Autodesk Inventor part; units mm, degrees
ref_plane "YZ Plane" through (0, 0, 0) normal (1, 0, 0) x (0, 1, 0)
ref_plane "XZ Plane" through (0, 0, 0) normal (0, 1, 0) x (-1, 0, 0)
ref_plane "Arbeitsebene1" through (0, 0, -17.5) normal (0, 0, 1) x (1, 0, 0)
sketch "Skizze1" plane through (0, 0, -17.5) normal (0, 0, 1) x (1, 0, 0)
  arc A0 (5.2, -17) -> (15.2, -17) centre (10.2, -17) ccw
  circle A1 centre (10.2, -17) radius 2.3
  circle A2 centre (10.2, 22) radius 2.3
  arc A3 (15.2, 22) -> (5.2, 22) centre (10.2, 22) ccw
  line L0 (15.2, 22) -> (15.2, -17)
  line L1 (5.2, -17) -> (5.2, 22)
  point P0 (0, 0)
  dimension "d17" = 39
  dimension "d19" = 5
  dimension "d20" = 5
  dimension "d21" = 4.6
  dimension "d22" = 4.6
  dimension "d23" = 5.2
  dimension "d24" = 15.2
  dimension "d25" = 17
extrude "Extrusion1" add sketch "Skizze1" against normal blind 20
sketch "Skizze2" plane through (15.2, -17, -17.5) normal (1, 0, 0) x (0, 0, -1)
  circle A0 centre (0.5, 19.5) radius 16
  circle A1 centre (0.5, 19.5) radius 19
  line L0 (0, 44) -> (20, 44)
  line L1 (7, 44) -> (7, 37.3536)
  line L2 (7, 44) -> (4.49, 46.4189)
  line L3 (4.49, 46.4189) -> (-2.5421, 44.7897)
  line L4 (-2.5421, 44.7897) -> (-3.0105, 35.1101)
  line L5 (-3.09, 3.908) -> (-10.3297, -18.857)
  line L6 (-10.3297, -18.857) -> (9.5227, -24.4173)
  line L7 (9.5227, -24.4173) -> (7, -5)
  line L8 (0, -5) -> (20, -5)
  line L9 (7, -5) -> (7, 1.6464)
  line L10 (0, 0) -> (0, -5)
  line L11 (36.0228, 70.8555) -> (-22.3921, 70.8555)
  line L12 (-22.3921, 70.8555) -> (-22.3921, -28.3632)
  line L13 (-22.3921, -28.3632) -> (36.0228, -28.3632)
  line L14 (36.0228, -28.3632) -> (36.0228, 70.8555)
  point P0 (-17.5, 17)
  point P1 (-4.0018, 1.041)
  point P2 (-2.861, 38.2004)
  dimension "d5" = 3
  dimension "d6" = 7
  dimension "d26" = 49
  dimension "d27" = 24.5
  dimension "d28" = 32
  dimension "d29" = 18
extrude "Extrusion2" cut sketch "Skizze2" against normal blind 10 contours A0 | L14 L13 L12 L11
sketch "Skizze3" plane through (15.2, -17, -24.5) normal (0, 0, -1) x (-1, 0, 0)
  circle A0 centre (5, 39) radius 2.3
  line L0 (2.8638, 35.3) -> (0.7276, 39)
  line L1 (0.7276, 39) -> (2.8638, 42.7)
  line L2 (2.8638, 42.7) -> (7.1362, 42.7)
  line L3 (7.1362, 42.7) -> (9.2724, 39)
  line L4 (9.2724, 39) -> (7.1362, 35.3)
  line L5 (7.1362, 35.3) -> (2.8638, 35.3)
  line L6 (0.7276, 0) -> (2.8638, 3.7)
  line L7 (2.8638, 3.7) -> (7.1362, 3.7)
  line L8 (7.1362, 3.7) -> (9.2724, 0)
  line L9 (9.2724, 0) -> (7.1362, -3.7)
  line L10 (7.1362, -3.7) -> (2.8638, -3.7)
  line L11 (2.8638, -3.7) -> (0.7276, 0)
  point P0 (15.2, 17)
  point P1 (5, 0)
  point P2 (5, 0)
  point P3 (5.6446, 34.7922)
  point P4 (4.3554, 34.7922)
  dimension "d9" = 7.4
  dimension "d10" = 7.4
extrude "Extrusion3" cut sketch "Skizze3" along normal blind 10 and the other way blind 3.5 contours A0 | L0 L1 L2 L3 L4 L5 | L6 L7 L8 L9 L10 L11
fillet "Rundung1" radius 1 2 edges at (15.2, 2.5, -37) (5.2, 2.5, -37)
equation "\"d20\" = d19"
equation "\"d27\" = 0.5 * d26"
equation "\"d10\" = d9"
properties part number "Schelle32"
Here's how the part is built. I have some questions about the finished solid (model axes, mm). A direction names the side the tool comes from. Give positions to 0.01 mm unless a question says otherwise; leave off trailing zeros. Loops run counter-clockwise (first coordinate to the right, second up) from the corner with the lowest first, then second, coordinate; pieces in that order, holes last. Notation, with made-up numbers: M -11,64 L 21,64 A29 cw 21,100 Z; hole C 79,-11.75 d7. An arc over 180 degrees is marked long. Use one line per item in the form item = value. Start each with the question number.
Q1. I need wall thicknesses on line 1 along Y through (x, z) = (10.2, -18.5); line 2 along Y through (x, z) = (10.2, -19.25); line 3 along Y through (x, z) = (10.5, -30.5). Which ranges of each line are inside material? Lowest first, please.
Q2. Which directions (+Z, -Z, +X, -X, +Y, -Y) give clear straight access to the entire face, cutting with the end or side of a thin tool? Please do faces 1 (the flat face through (8, 24, -21)), 2 (the flat face through (15.2, 2.6, -34.2)).
Q3. If we section it at C-C (y = 2.5): Write out the boundary of the cut face in (x, z), then the cut area to 3 significant figures.
Q4. If we section it at D-D (x = 13): Write out the boundary of the cut face in (y, z).
Q5. Will these pins go through, and if not, where does the flat tip stop? pin 1 Ø4 at (x, y) = (9, 24.5) entering from -Z; pin 2 Ø6 at (x, z) = (14, -24) entering from +Y; pin 3 Ø2 at (y, z) = (12, -29) entering from +X; pin 4 Ø3.5 at (x, y) = (8, 21) entering from -Z.
Q6. If we section it at B-B (z = -20.25): Write out the boundary of the cut face in (x, y), then the cut area to 3 significant figures.
Taken from the geometry:
q1.line_1 = -22 to -19.3, -14.7 to -13.49, 18.49 to 19.7, 24.3 to 27
q1.line_2 = -22 to -19.3, -14.7 to -13.45, 18.45 to 19.7, 24.3 to 27
q1.line_3 = -11.81 to -7.49, 12.49 to 16.81
q2.face_1 = -Z
q2.face_2 = +Z, -Z, +X, +Y, -Y
q3.outline = M 5.2,-36 A1 ccw 6.2,-37 L 14.2,-37 A1 ccw 15.2,-36 L 15.2,-34 L 5.2,-34 Z
q3.area = 29.6 mm^2
q4.outline = M -21.14,-24.5 L -19.55,-24.5 L -19.55,-21 L -14.45,-21 L -14.45,-26.59 A19 ccw 19.45,-26.59 L 19.45,-21 L 24.55,-21 L 24.55,-24.5 L 26.14,-24.5 L 26.14,-17.5 L 18.49,-17.5 A16 cw long -13.49,-17.5 L -21.14,-17.5 Z
q5.pin_1 = -24.5
q5.pin_2 = 26.94
q5.pin_3 = through
q5.pin_4 = -26.81
q6.outline = M 5.2,-17 A5 ccw 15.2,-17 L 15.2,-13.34 L 5.2,-13.34 Z; M 5.2,18.34 L 15.2,18.34 L 15.2,22 A5 ccw 5.2,22 Z; hole C 10.2,-17 d4.6; hole C 10.2,22 d4.6
q6.area = 118 mm^2
